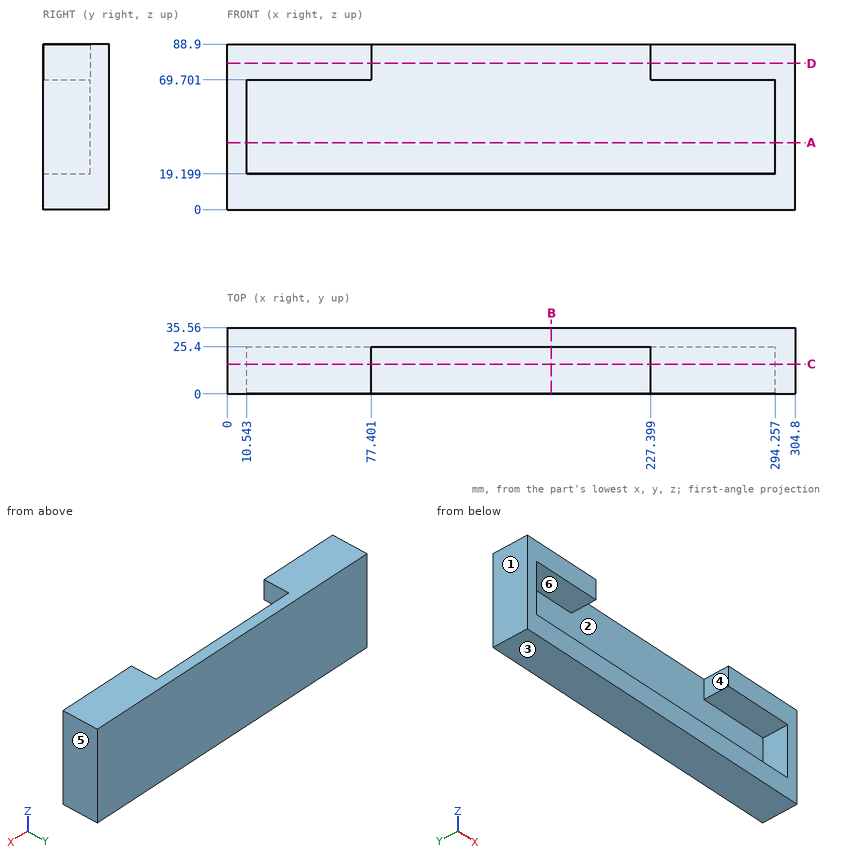
Drawing for the job (mm, zero at the part's lowest x, y, z). A direction names the side the tool comes from. Give positions to 0.01 mm unless a question says otherwise; leave off trailing zeros. Write each loop counter-clockwise with the first axis right and the second up, starting at its lowest first coordinate (ties: lowest second). Pieces come first, ordered by that corner, then holes. Notation, with made-up numbers: M 26,36.25 L 68,36.25 A33 cw 68,64.25 Z; hole C -6,13.25 d10. An arc over 180 degrees is marked long. Return JSON: item names as keys, results as strings. Group by question number.
(1) Band-saw the part on A-A (z = 36). Give the cut face in (x, y).
(2) Flat gauge pins, fed straight in: pin 1 Ø2 at (x, y) = (118, 21.5) entering from -Z; pin 2 Ø20.5 at (x, y) = (92, 8) entering from +Z; pin 3 Ø21 at (x, z) = (180, 71) entering from -Y. Where does each tip first touch, or does it go through?
(3) Band-saw the part on B-B (x = 174). Give the cut face in (y, z).
(4) 3-axis set-ups, long thin cutter, end or side, ignore diameter. For the marked faces 4, 5 and 6: which of +Z, -Z, +X, -X, +Y, -Y reach the whole face in a straight line?
(5) Mould opens along X. For the marked faces 1, 2 and 3 say: pulls with the +X half, pulls with the -X half, needs draft (parallel to the pull), parting line crosses it, or undercut.
(6) Drill centre lines: L1, parallel to Z at x = 34, y = 6.5; L2, parallel to X at y = 13.5, z = 56.5; L3, parallel to Z at x = 172.5, y = 12. Where is each one in solid material? Low to high. Write a range as [from, to].
(7) Band-saw the part on C-C (y = 16). Give the cut face in (x, z), and give its area (3 significant figures).
(8) Band-saw the part on D-D (z = 78.5). Give the cut face in (x, y).
Entries:
{
 "1": {"outline": "M 0,0 L 10.54,0 L 10.54,25.4 L 294.26,25.4 L 294.26,0 L 304.8,0 L 304.8,35.56 L 0,35.56 Z"},
 "2": {"pin 1": "stops at z = 0", "pin 2": "stops at z = 19.2", "pin 3": "stops at y = 25.4"},
 "3": {"outline": "M 0,0 L 35.56,0 L 35.56,88.9 L 25.4,88.9 L 25.4,19.2 L 0,19.2 Z"},
 "4": {"face 4": "+Z, -Y", "face 5": "+Z, -Z, +X, +Y, -Y", "face 6": "-Y"},
 "5": {"face 1": "pulls with the -X half", "face 2": "undercut", "face 3": "needs draft"},
 "6": {"L1": "z = [0, 19.2], [69.7, 88.9]", "L2": "x = [0, 10.54], [294.26, 304.8]", "L3": "z = [0, 19.2]"},
 "7": {"outline": "M 0,0 L 304.8,0 L 304.8,88.9 L 227.4,88.9 L 227.4,69.7 L 294.26,69.7 L 294.26,19.2 L 10.54,19.2 L 10.54,69.7 L 77.4,69.7 L 77.4,88.9 L 0,88.9 Z", "area": "9,890 mm^2"},
 "8": {"outline": "M 0,0 L 77.4,0 L 77.4,25.4 L 227.4,25.4 L 227.4,0 L 304.8,0 L 304.8,35.56 L 0,35.56 Z"}
}
